Autodesk Inventor part; units mm, degrees
ref_plane "YZ Plane" through (0, 0, 0) normal (1, 0, 0) x (0, 1, 0)
ref_plane "XZ Plane" through (0, 0, 0) normal (0, 1, 0) x (-1, 0, 0)
ref_plane "XY Plane" through (0, 0, 0) normal (0, 0, 1) x (1, 0, 0)
sketch "Sketch1" plane through (0, 0, 0) normal (0, 1, 0) x (-1, 0, 0)
  line L0 (0, 0) -> (-20, 0)
  line L1 (-20, 0) -> (-20, 20)
  line L2 (-20, 20) -> (0, 20)
  line L3 (0, 20) -> (0, 0)
  line L4 (-20, 20) -> (-4, 20)
  line L5 (-4, 20) -> (-4, 4)
  line L6 (-4, 4) -> (-20, 4)
  line L7 (-20, 4) -> (-20, 20)
  dimension "d0" = 20
  dimension "d1" = 20
  dimension "d2" = 16
  dimension "d3" = 16
extrude "Extrusion1" add sketch "Sketch1" along normal blind 20 contours L0 L1 L6 L5 L2 L3
sketch "Sketch2" plane through (0, 0, 0) normal (-1, 0, 0) x (0, 0, 1)
  line L0 (0, 0) -> (10, 0)
  line L1 (10, 0) -> (10, 10)
  line L2 (10, 10) -> (0, 10)
  line L3 (0, 10) -> (0, 0)
  circle A0 centre (10, 10) radius 2.5
  dimension "d6" = 10
  dimension "d7" = 10
  dimension "d8" = 5
extrude "Extrusion2" cut sketch "Sketch2" against normal blind 20 contours A0 L2 L1 | L1 L2 A0
sketch "Sketch3" plane through (20, 0, 0) normal (0, 0, -1) x (-1, 0, 0)
  line L0 (16, 0) -> (0, 0)
  line L1 (0, 0) -> (5, 0)
  line L2 (5, 0) -> (5, 10)
  line L3 (5, 10) -> (0, 10)
  line L4 (0, 10) -> (0, 0)
  circle A0 centre (5, 10) radius 2.5
  point P0 (20, 0)
  dimension "d11" = 5
  dimension "d12" = 10
  dimension "d13" = 5
extrude "Extrusion3" cut sketch "Sketch3" against normal blind 20 contours A0 L3 L2 | L2 L3 A0
sketch "Sketch4" plane through (20, 0, 4) normal (1, 0, 0) x (0, 0, -1)
  line L0 (4, 0) -> (-16, 0)
  line L1 (0, 0) -> (0, 20)
  line L2 (4, 0) -> (0, 0)
  line L3 (0, 0) -> (0, 20)
  line L4 (0, 20) -> (4, 20)
  line L5 (4, 20) -> (4, 0)
extrude "Extrusion4" add sketch "Sketch4" along normal blind 7
properties part number "l-holder_2020"
Check sheet for the modelled part. Datum: model origin and axes. Units: mm. A direction names the side the tool comes from. Coordinates: 2 decimals unless noted, no trailing zeros. Write each loop counter-clockwise with the first axis right and the second up, starting at its lowest first coordinate (ties: lowest second). Pieces come first, ordered by that corner, then holes.
Item 1: Cross-section at C-C on z = 10. Record the boundary of the cut face in (x, y), then the cut area to 3 significant figures.
Numbers:
outline: (0, 0) - (4, 0) - (4, 7.5) - (0, 7.5) - close; (0, 12.5) - (4, 12.5) - (4, 20) - (0, 20) - close
area: 60.0 mm2
Item 2: Mould release check, pull along Z, two halves, no side actions. Record for faces 3 (the face through (13, 12, 0)), 4 (the face through (0, 8, 12)), 5 (the face through (18, 10, 4)), 6 (the face through (1.97, 7.56, 9.46)): released by +Z, released by -Z, zero draft, split by the parting line, or undercut.
Numbers:
face 3: released by -Z
face 4: zero draft
face 5: released by +Z
face 6: undercut
Item 3: Depth check by flat-ended pin: pin 1 Ø1 at (x, y) = (18, 9.5) entering from +Z; pin 2 Ø5 at (y, z) = (11, 10) entering from +X. Enter the tip coordinate at first touch or a pass-through.
Numbers:
pin 1: stops at z = 4
pin 2: stops at x = 4
Item 4: Cross-section at D-D on y = 19.25. Record the boundary of the cut face in (x, z).
Numbers:
outline: (0, 0) - (27, 0) - (27, 4) - (4, 4) - (4, 20) - (0, 20) - close
Item 5: Scan lines: probe 1 along Y at (x, z) = (15, 0.8); probe 2 along Z at (x, y) = (16, 3). Record each from-to range of solid material in increasing order.
Numbers:
probe 1: y = 0 to 7.5, 12.5 to 20
probe 2: z = 0 to 4
Item 6: Cross-section at A-A on x = 15. Record the boundary of the cut face in (y, z).
Numbers:
outline: (0, 0) - (7.5, 0) - (7.5, 4) - (0, 4) - close; (12.5, 0) - (20, 0) - (20, 4) - (12.5, 4) - close
Item 7: Cross-section at B-B on y = 10. Record the boundary of the cut face in (x, z), then the cut area to 3 significant figures.
Numbers:
outline: (0, 0) - (12.5, 0) - (12.5, 4) - (4, 4) - (4, 7.5) - (0, 7.5) - close; (0, 12.5) - (4, 12.5) - (4, 20) - (0, 20) - close; (17.5, 0) - (27, 0) - (27, 4) - (17.5, 4) - close
area: 132 mm2
Item 8: Access from +Z, -Z, +X, -X, +Y, -Y to the whole of each face (thin tool, end or side, straight path). Record for faces 1 (the face through (10, 0, 3)), 2 (the face through (4, 10, 14)).
Numbers:
face 1: +Z, -Z, +X, -X, -Y
face 2: +Z, +X, +Y, -Y
